Read the model definition and answer for the solid it produces. Units are mm, in the model's axes. Coordinates: 2 decimals unless noted, no trailing zeros. Order: outer loops, then holes, each group sorted by start corner. A loop starts at its lowest first (then second) coordinate and runs counter-clockwise, first axis right, second up. Notation, with made-up numbers: M -19,32.25 L 21,32.25 A16 cw 21,56.25 Z; hole C 2.25,12.5 d7. An arc over 180 degrees is marked long. Use a Markdown table: item, result. Add a question column.
1) Find section D-D on z = -4. Write down the section's boundary in (x, y).
2) Find section C-C on x = 0. Write down the section's boundary in (y, z).
3) Find the intervals of material crossed by probe 1 along Z at (x, y) = (0, -0.4); probe 2 along X at (y, z) = (1, -1); probe 3 along Y at (x, z) = (5.25, 3), in increasing order. Write a range as [from, to].
4) Find section A-A on y = 1. Write down the section's boundary in (x, z), plus the area to 3 significant figures.
5) Each of these flat-tipped pins is pushed along its axis until it touches: pin 1 Ø1 at (x, y) = (6.5, 2) entering from +Z; pin 2 Ø5.5 at (x, z) = (3, -9) entering from +Y; pin 3 Ø0.8 at (y, z) = (-0.5, -16.5) entering from +X; pin 4 Ø7 at (x, z) = (0, -13) entering from -Y. Where does it stop, or does it pass through?
6) Find section B-B on z = 13. Write down the section's boundary in (x, y), plus the area to 3 significant figures.
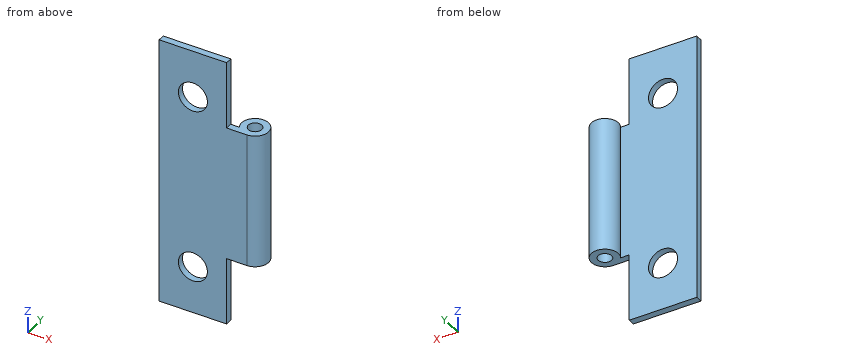
from build123d import *

# Parameters (mm, degrees)
F0_W     = 3
F0_H     = 20
F1_DEPTH = 1
F2_W     = 1
F2_H     = 20
F5_D     = 4.3
F5_DEPTH = 2.5
F5_TIP   = 1.2918503309


# Not quite as in the source:
# - a feature names something its author has since deleted; it is built from what else it names


with BuildPart() as f1:
    # F0 (on Front) → F1 (new body)
    with BuildSketch(Plane.XZ):
        Polygon((5, 10), (5, 20), (-5, 20), (-5, -20), (5, -20), (5, -10), align=None)
        with Locations((6.5, 0)):
            Rectangle(F0_W, F0_H)
    extrude(amount=F1_DEPTH)

    # F2 (on face) → F3 (revolve)
    with BuildSketch(Plane.YZ.offset(8)):
        with Locations((-0.5, 0)):
            Rectangle(F2_W, F2_H)
    revolve(axis=Axis((8, 1, 0), (0, 0, 1)))

    # F5
    with Locations(Plane.XZ.offset(1)):
        with Locations((0, 13), (0, -13)):
            Hole(F5_D / 2, depth=F5_DEPTH)
            with Locations((0, 0, -(F5_DEPTH + F5_TIP / 2))):  # 118° drill point
                Cone(0, F5_D / 2, F5_TIP, mode=Mode.SUBTRACT)


solid = f1.part
Check result:
| question | item | result |
|---|---|---|
| 1 | outline | M -5,-1 L 8,-1 A2 ccw long 6.27,0 L -5,0 Z; hole C 8,1 d2 |
| 2 | outline | M -1,-20 L 0,-20 L 0,-15.15 L -1,-15.15 Z; M -1,-10.85 L 0,-10.85 L 0,10.85 L -1,10.85 Z; M -1,15.15 L 0,15.15 L 0,20 L -1,20 Z |
| 3 | probe 1 | z = [-20, -15.15], [-10.85, 10.85], [15.15, 20] |
| 3 | probe 2 | x = [6, 7], [9, 10] |
| 3 | probe 3 | y = [-1, 0] |
| 4 | outline | M 6,-10 L 7,-10 L 7,10 L 6,10 Z; M 9,-10 L 10,-10 L 10,10 L 9,10 Z |
| 4 | area | 40.0 mm2 |
| 5 | pin 1 | stops at z = 10 |
| 5 | pin 2 | stops at y = 0 |
| 5 | pin 3 | stops at x = 5 |
| 5 | pin 4 | stops at y = -1 |
| 6 | outline | M -5,-1 L -2.15,-1 L -2.15,0 L -5,0 Z; M 2.15,-1 L 5,-1 L 5,0 L 2.15,0 Z |
| 6 | area | 5.70 mm2 |
